Design review of the part built by this model. Coordinates are the model's own, in mm. Face numbers are marked on the shaded views. Coordinates: 2 decimals unless noted, no trailing zeros. Write each loop counter-clockwise with the first axis right and the second up, starting at its lowest first coordinate (ties: lowest second). Pieces come first, ordered by that corner, then holes. Notation, with made-up numbers: (52.25, -17.75) - (71.25, -17.75) arc R12 ccw to (71.25, -13.75) - close; hole circle Ø9 at (30.25, 31.5). An arc over 180 degrees is marked (long way). Answer as a JSON object with one key per item and string values.
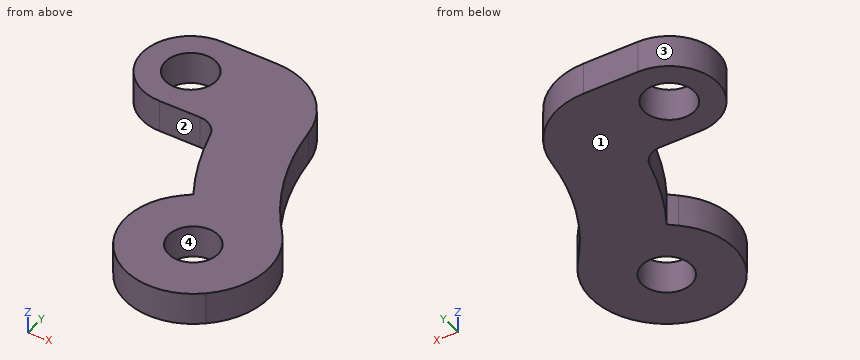
```python
from build123d import *

# Parameters (mm, degrees)
SKETCH1_R           = 2.35
SKETCH1_R_2         = 2.3
BOSS_EXTRUDE2_DEPTH = 3


with BuildPart() as part:
    # Sketch1 → Boss-Extrude2 (new body)
    with BuildSketch(Plane.XY.offset(-130.24387898)):
        with BuildLine():
            Line((-15.010059364, 38.189351968), (-15.708117617, 37.572463316))
            ThreePointArc((-15.708117617, 37.572463316), (-16.257044738, 28.67984396), (-7.364425381, 28.130916839))
            Line((-7.364425381, 28.130916839), (-7.27434556, 28.210522262))
            ThreePointArc((-7.27434556, 28.210522262), (-4.930575043, 32.916016457), (-6.522896429, 37.925951432))
            ThreePointArc((-6.522896429, 37.925951432), (-9.929258204, 43.436995693), (-11.691880866, 49.671421949))
            ThreePointArc((-11.691880866, 49.671421949), (-14.02608552, 53.994717475), (-18.626779298, 55.718960016))
            Line((-18.626779298, 55.718960016), (-23.716053845, 55.718960016))
            ThreePointArc((-23.716053845, 55.718960016), (-28.216053845, 51.218960016), (-23.716053845, 46.718960016))
            Line((-23.716053845, 46.718960016), (-19.942226175, 46.718960016))
            ThreePointArc((-19.942226175, 46.718960016), (-18.729620599, 46.309427783), (-18.013616093, 45.248547734))
            ThreePointArc((-18.013616093, 45.248547734), (-16.74918621, 41.617962479), (-15.010059364, 38.189351968))
        make_face()
        with Locations((-23.716053845, 51.218960016)):
            Circle(SKETCH1_R, mode=Mode.SUBTRACT)
        with Locations((-11.536271499, 32.851690078)):
            Circle(SKETCH1_R_2, mode=Mode.SUBTRACT)
    extrude(amount=BOSS_EXTRUDE2_DEPTH)


solid = part.part
```
(1) To check wall thickness, follow line 1 (X direction, y = 31.25, z = -128.9); line 2 (X direction, y = 52.25, z = -128.6); line 3 (Y direction, x = -12.5, z = -129.4). State the ranges of each line that lie inside material, in increasing order. Write a range as from..to.
Solved:
{"line 1": "x = -17.63..-13.19, -9.89..-5.27", "line 2": "x = -28.1..-25.83, -21.6..-12.58", "line 3": "y = 26.63..30.76, 34.94..52.1"}
(2) Take a section at D-D, the plane y = 41. Write out the cut boundary in (x, z), and give its area (3 significant figures).
Solved:
{"outline": "(-16.48, -130.24) - (-8.68, -130.24) - (-8.68, -127.24) - (-16.48, -127.24) - close", "area": "23.4 mm^2"}
(3) For pin 1 (1.5 mm diameter, centred on y = 33.5, z = -128, fed in from -X); pin 2 (4 mm diameter, centred on x = -21, y = 46.5, fed in from +Z); pin 3 (1.5 mm diameter, centred on x = -9, z = -128.5, fed in from +Y), all flat-tipped, find the tip position at first contact; note any pin that passes through.
Solved:
{"pin 1": "stops at x = -17.84", "pin 2": "stops at z = -127.24", "pin 3": "stops at y = 43.04"}
(4) Take a section at B-B, the plane y = 52.75. Write out the cut boundary in (x, z).
Solved:
{"outline": "(-27.95, -130.24) - (-25.5, -130.24) - (-25.5, -127.24) - (-27.95, -127.24) - close; (-21.93, -130.24) - (-12.9, -130.24) - (-12.9, -127.24) - (-21.93, -127.24) - close"}
(5) Take a section at A-A, the plane x = -17.25. Write out the cut boundary in (y, z), and give its area (3 significant figures).
Solved:
{"outline": "(30.2, -130.24) - (35.51, -130.24) - (35.51, -127.24) - (30.2, -127.24) - close; (42.88, -130.24) - (55.58, -130.24) - (55.58, -127.24) - (42.88, -127.24) - close", "area": "54.0 mm^2"}
(6) Take a section at C-C, the plane z = -129.4. Write out the cut boundary in (x, y).
Solved:
{"outline": "(-23.72, 46.72) - (-19.94, 46.72) arc R2 cw to (-18.01, 45.25) arc R28.65 ccw to (-15.01, 38.19) - (-15.71, 37.57) arc R6.3 ccw to (-7.36, 28.13) - (-7.27, 28.21) arc R7 ccw to (-6.52, 37.93) arc R23.37 cw to (-11.69, 49.67) arc R7 ccw to (-18.63, 55.72) - (-23.72, 55.72) arc R4.5 ccw to start; hole circle Ø4.7 at (-23.72, 51.22); hole circle Ø4.6 at (-11.54, 32.85)"}
(7) The part is to be moulded in two halves that separate along Y. For the marked faces 1, 2, 3 and 4, say which applies: pulls with the +Y half, pulls with the -Y half, needs draft (parallel to the pull), parting line crosses it, or undercut.
Solved:
{"face 1": "needs draft", "face 2": "pulls with the -Y half", "face 3": "parting line crosses it", "face 4": "undercut"}
